Design review of the part shown in the three views and the two pictorial views. Dimensions are in mm from the part's minimum x, y and z. Give positions to 0.01 mm unless a question says otherwise; leave off trailing zeros. Order: outer loops, then holes, each group sorted by start corner. A loop starts at its lowest first (then second) coordinate and runs counter-clockwise, first axis right, second up.
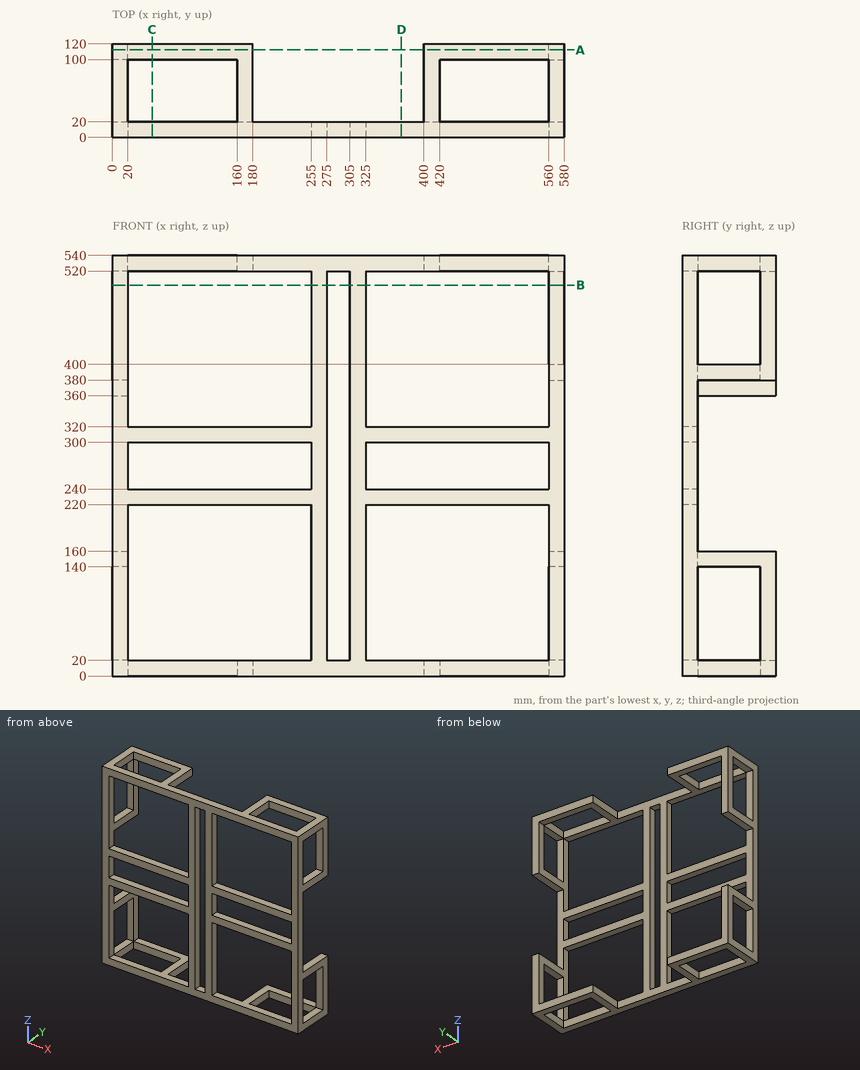
Item 1: For line 1 (Z direction, x = 332, y = 16); line 2 (X direction, y = 13, z = 202); line 3 (Z direction, x = 515.5, y = 114), list the stretches that pass through material, from the lowest coordinate up.
Values found:
line 1: z = 0 to 20, 220 to 240, 300 to 320, 520 to 540
line 2: x = 0 to 20, 255 to 275, 305 to 325, 560 to 580
line 3: z = 0 to 20, 520 to 540
Item 2: Take a section at C-C (x = 51). Give the boundary of the cut face in (y, z), and give its area (3 significant figures).
Values found:
outline: (0, 0) - (20, 0) - (20, 20) - (0, 20) - close; (0, 220) - (20, 220) - (20, 240) - (0, 240) - close; (0, 300) - (20, 300) - (20, 320) - (0, 320) - close; (0, 520) - (20, 520) - (20, 540) - (0, 540) - close; (100, 0) - (120, 0) - (120, 20) - (100, 20) - close; (100, 520) - (120, 520) - (120, 540) - (100, 540) - close
area: 2,400 mm2
Item 3: Take a section at D-D (x = 371). Give the boundary of the cut face in (y, z).
Values found:
outline: (0, 0) - (20, 0) - (20, 20) - (0, 20) - close; (0, 220) - (20, 220) - (20, 240) - (0, 240) - close; (0, 300) - (20, 300) - (20, 320) - (0, 320) - close; (0, 520) - (20, 520) - (20, 540) - (0, 540) - close
Item 4: Take a section at B-B (z = 502). Give the boundary of the cut face in (x, y), and give its area (3 significant figures).
Values found:
outline: (0, 0) - (20, 0) - (20, 20) - (0, 20) - close; (0, 100) - (20, 100) - (20, 120) - (0, 120) - close; (255, 0) - (275, 0) - (275, 20) - (255, 20) - close; (305, 0) - (325, 0) - (325, 20) - (305, 20) - close; (560, 0) - (580, 0) - (580, 20) - (560, 20) - close; (560, 100) - (580, 100) - (580, 120) - (560, 120) - close
area: 2,400 mm2
Item 5: Take a section at A-A (y = 112.5). Give the boundary of the cut face in (x, z).
Values found:
outline: (0, 0) - (180, 0) - (180, 20) - (20, 20) - (20, 160) - (0, 160) - close; (0, 360) - (20, 360) - (20, 520) - (180, 520) - (180, 540) - (0, 540) - close; (400, 0) - (580, 0) - (580, 160) - (560, 160) - (560, 20) - (400, 20) - close; (400, 520) - (560, 520) - (560, 380) - (580, 380) - (580, 540) - (400, 540) - close
